from build123d import *

# Parameters (mm, degrees)
SKETCH1_W                  = 25.4
SKETCH1_H                  = 1498.6
BOSS_EXTRUDE1_DEPTH        = 25.4
SKETCH2_W                  = 23.114
SKETCH2_H                  = 23.114
CUT_EXTRUDE1_DEPTH         = 1499.6
M3_5_CLEARANCE_HOLE1_D     = 4.1402
M3_5_CLEARANCE_HOLE1_DEPTH = 25.4
M3_5_CLEARANCE_HOLE2_D     = 4.1402
M3_5_CLEARANCE_HOLE2_DEPTH = 25.4
CHAMFER1_SIZE              = 2.159
FILLET1_R                  = 0.8128
FILLET2_R                  = 3.0988
SKETCH8_W                  = 95.882963774
SKETCH8_H                  = 79.338329604
CUT_EXTRUDE3_DEPTH         = 1371.6
SKETCH11_W                 = 51.462522779
SKETCH11_H                 = 66.676735099
CUT_EXTRUDE6_DEPTH         = 2.286
SKETCH12_W                 = 24.634530663
SKETCH12_H                 = 66.668992962
CUT_EXTRUDE7_DEPTH         = 2.54


with BuildPart() as part:
    # Sketch1 → Boss-Extrude1 (new body)
    with BuildSketch(Plane(origin=(0, 0, 0), x_dir=(0, -1, 0), z_dir=(-1, 0, 0))):
        with Locations((-12.7, 0)):
            Rectangle(SKETCH1_W, SKETCH1_H)
    extrude(amount=-BOSS_EXTRUDE1_DEPTH)

    # Sketch2 → Cut-Extrude1 (cut, through all)
    with BuildSketch(Plane(origin=(0, 0, -749.3), x_dir=(-1, 0, 0), z_dir=(0, 0, -1))):
        with Locations((-13.843, 13.843)):
            Rectangle(SKETCH2_W, SKETCH2_H)
    extrude(amount=-CUT_EXTRUDE1_DEPTH, mode=Mode.SUBTRACT)

    # M3.5 Clearance Hole1
    with Locations(Plane(origin=(0, 0, 0), x_dir=(-1, 0, 0), z_dir=(0, -1, 0))):
        with Locations((-12.7, 736.6), (-12.7, 711.2), (-12.7, 685.8), (-12.7, 660.4), (-12.7, 635), (-12.7, 609.6), (-12.7, 584.2), (-12.7, 558.8), (-12.7, 533.4), (-12.7, 508), (-12.7, 482.6), (-12.7, 457.2), (-12.7, 431.8), (-12.7, 406.4), (-12.7, 381), (-12.7, 355.6), (-12.7, 330.2), (-12.7, 304.8), (-12.7, 279.4), (-12.7, 254), (-12.7, 228.6), (-12.7, 203.2), (-12.7, 177.8), (-12.7, 152.4), (-12.7, 127), (-12.7, 101.6), (-12.7, 76.2), (-12.7, 50.8), (-12.7, 25.4), (-12.7, 0), (-12.7, -25.4), (-12.7, -50.8), (-12.7, -76.2), (-12.7, -101.6), (-12.7, -127), (-12.7, -152.4), (-12.7, -177.8), (-12.7, -203.2), (-12.7, -228.6), (-12.7, -254), (-12.7, -279.4), (-12.7, -304.8), (-12.7, -330.2), (-12.7, -355.6), (-12.7, -381), (-12.7, -406.4), (-12.7, -431.8), (-12.7, -457.2), (-12.7, -482.6), (-12.7, -508), (-12.7, -533.4), (-12.7, -558.8), (-12.7, -584.2), (-12.7, -609.6), (-12.7, -635), (-12.7, -660.4), (-12.7, -685.8), (-12.7, -711.2), (-12.7, -736.6)):
            Hole(M3_5_CLEARANCE_HOLE1_D / 2, depth=M3_5_CLEARANCE_HOLE1_DEPTH)

    # M3.5 Clearance Hole2
    with Locations(Plane.ZY):
        with Locations((711.2, 12.7), (736.6, 12.7), (685.8, 12.7), (660.4, 12.7), (635, 12.7), (609.6, 12.7), (584.2, 12.7), (558.8, 12.7), (533.4, 12.7), (508, 12.7), (482.6, 12.7), (457.2, 12.7), (431.8, 12.7), (406.4, 12.7), (381, 12.7), (355.6, 12.7), (330.2, 12.7), (304.8, 12.7), (279.4, 12.7), (254, 12.7), (228.6, 12.7), (203.2, 12.7), (177.8, 12.7), (152.4, 12.7), (127, 12.7), (101.6, 12.7), (76.2, 12.7), (50.8, 12.7), (25.4, 12.7), (0, 12.7), (-25.4, 12.7), (-50.8, 12.7), (-76.2, 12.7), (-101.6, 12.7), (-127, 12.7), (-152.4, 12.7), (-177.8, 12.7), (-203.2, 12.7), (-228.6, 12.7), (-254, 12.7), (-279.4, 12.7), (-304.8, 12.7), (-330.2, 12.7), (-355.6, 12.7), (-381, 12.7), (-406.4, 12.7), (-431.8, 12.7), (-457.2, 12.7), (-482.6, 12.7), (-508, 12.7), (-533.4, 12.7), (-558.8, 12.7), (-584.2, 12.7), (-609.6, 12.7), (-635, 12.7), (-660.4, 12.7), (-685.8, 12.7), (-711.2, 12.7), (-736.6, 12.7)):
            Hole(M3_5_CLEARANCE_HOLE2_D / 2, depth=M3_5_CLEARANCE_HOLE2_DEPTH)

    # Chamfer1
    chamfer1_edges = [part.edges().sort_by_distance(p)[0] for p in [
        (25.4, 1.143, -749.3),
        (1.143, 25.4, 749.3),
        (1.143, 25.4, -749.3),
        (25.4, 1.143, 749.3),
    ]]
    chamfer(chamfer1_edges, length=CHAMFER1_SIZE)

    # Fillet1
    fillet1_edges = [part.edges().sort_by_distance(p)[0] for p in [
        (2.286, 2.286, 0),
    ]]
    fillet(fillet1_edges, radius=FILLET1_R)

    # Fillet2
    fillet2_edges = [part.edges().sort_by_distance(p)[0] for p in [
        (0, 0, 0),
    ]]
    fillet(fillet2_edges, radius=FILLET2_R)

    # Sketch8 → Cut-Extrude3 (cut)
    with BuildSketch(Plane.XY.offset(749.3)):
        with Locations((2.286, 3.0988)):
            Rectangle(SKETCH8_W, SKETCH8_H)
    extrude(amount=-CUT_EXTRUDE3_DEPTH, mode=Mode.SUBTRACT)

    # Sketch11 → Cut-Extrude6 (cut)
    with BuildSketch(Plane.XY.offset(-622.3)):
        with Locations((1.85517497, 1.74884985)):
            Rectangle(SKETCH11_W, SKETCH11_H)
    extrude(amount=-CUT_EXTRUDE6_DEPTH, mode=Mode.SUBTRACT)

    # Sketch12 → Cut-Extrude7 (cut)
    with BuildSketch(Plane(origin=(0, 2.286, 0), x_dir=(1, 0, 0), z_dir=(0, 1, 0))):
        with Locations((15.416065332, 719.134496481)):
            Rectangle(SKETCH12_W, SKETCH12_H)
    extrude(amount=-CUT_EXTRUDE7_DEPTH, mode=Mode.SUBTRACT)


solid = part.part
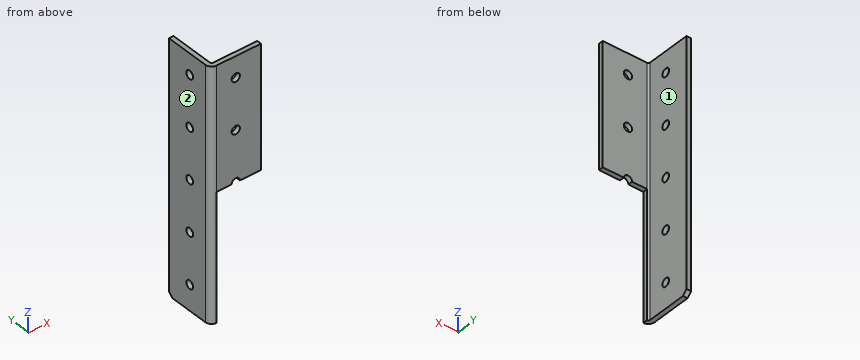
CAD build for the part. Positions are in the model's coordinates, mm. Face numbers are marked on the shaded views. A direction names the side the tool comes from. Give positions to 0.01 mm unless a question says otherwise; leave off trailing zeros. Order: outer loops, then holes, each group sorted by start corner. A loop starts at its lowest first (then second) coordinate and runs counter-clockwise, first axis right, second up. Notation, with made-up numbers: (71, -18) - (95, -18) arc R23 ccw to (95, 20) - close; hole circle Ø9 at (89, -9). An arc over 180 degrees is marked (long way). Answer in a Markdown table with one row per item.
1. Saw through at B-B, the plane z = -711.2. Give the cut face in (x, y).
Data:
| item | result |
|---|---|
| outline | (0, 3.1) arc R3.1 ccw to (3.1, 0) - (3.1, 2.29) arc R0.81 cw to (2.29, 3.1) - (2.29, 10.63) - (0, 10.63) - close; (0, 14.77) - (2.29, 14.77) - (2.29, 25.4) - (0, 25.4) - close |
2. Saw through at A-A, the plane z = -660.4. Give the cut face in (x, y), plus the area to 3 significant figures.
Data:
| item | result |
|---|---|
| outline | (0, 3.1) arc R3.1 ccw to (3.1, 0) - (10.63, 0) - (10.63, 2.29) - (3.1, 2.29) arc R0.81 cw to (2.29, 3.1) - (2.29, 10.63) - (0, 10.63) - close; (0, 14.77) - (2.29, 14.77) - (2.29, 25.4) - (0, 25.4) - close; (14.77, 0) - (25.4, 0) - (25.4, 2.29) - (14.77, 2.29) - close |
| area | 90.1 mm² |
3. Probe probe 1 along Z at (x, y) = (12.7, 1.7); probe 2 along Y at (x, z) = (14.5, -633); probe 3 along Y at (x, z) = (1.45, -635). List the from-to ranges inside material, lowest first. Write a range as [from, to].
Data:
| item | result |
|---|---|
| probe 1 | z = [-683.73, -662.47], [-658.33, -637.07], [-632.93, -624.59] |
| probe 2 | y = [0, 2.29] |
| probe 3 | y = [0.48, 10.63], [14.77, 25.4] |
4. Tool access for the marked faces 1 and 2: list every direction of +Z, -Z, +X, -X, +Y, -Y with a clear straight run to the whole face (end or side of a thin tool).
Data:
| item | result |
|---|---|
| face 1 | +Z, -Z, +X, +Y |
| face 2 | +Z, -Z, -X, +Y, -Y |
5. Saw through at D-D, the plane x = 12.75. Give the cut face in (y, z).
Data:
| item | result |
|---|---|
| outline | (0, -683.73) - (2.29, -683.73) - (2.29, -662.47) - (0, -662.47) - close; (0, -658.33) - (2.29, -658.33) - (2.29, -637.07) - (0, -637.07) - close; (0, -632.93) - (2.29, -632.93) - (2.29, -624.59) - (0, -624.59) - close |
6. Flat gauge pins, fed straight in: pin 1 (0.7 mm diameter, centred on x = 7.5, y = 0.5, fed in from -Z); pin 2 (5 mm diameter, centred on x = 5, z = -706.5, fed in from +Y); pin 3 (6 mm diameter, centred on y = 19, z = -645.5, fed in from +X). Where does each tip first touch, or does it go through?
Data:
| item | result |
|---|---|
| pin 1 | stops at z = -685.8 |
| pin 2 | stops at y = 2.55 |
| pin 3 | stops at x = 2.29 |
7. Saw through at C-C, the plane y = 12.7. Give the cut face in (x, z).
Data:
| item | result |
|---|---|
| outline | (0, -749.3) - (2.29, -749.3) - (2.29, -738.67) - (0, -738.67) - close; (0, -734.53) - (2.29, -734.53) - (2.29, -713.27) - (0, -713.27) - close; (0, -709.13) - (2.29, -709.13) - (2.29, -687.87) - (0, -687.87) - close; (0, -683.73) - (2.29, -683.73) - (2.29, -662.47) - (0, -662.47) - close; (0, -658.33) - (2.29, -658.33) - (2.29, -637.07) - (0, -637.07) - close; (0, -632.93) - (2.29, -632.93) - (2.29, -624.59) - (0, -624.59) - close |
